CAD build for the part. Positions are in the model's coordinates, mm. A direction names the side the tool comes from. Give positions to 0.01 mm unless a question says otherwise; leave off trailing zeros. Loops run counter-clockwise (first coordinate to the right, second up) from the corner with the lowest first, then second, coordinate; pieces in that order, holes last. Notation, with made-up numbers: M 7.25,28.25 L 51.25,28.25 A27 ccw 51.25,56.25 Z; hole C 18.5,89 d6. An arc over 180 degrees is marked long. One line per question, with ' | ' between items.
Autodesk Inventor part; units mm, degrees
ref_plane "Work Plane2" through (0, 0, 2.5) normal (0, 0, 1) x (1, 0, 0)
ref_plane "Work Plane8" through (0, 0, 0) normal (0.9238795, 0.3826834, 0) x (0, 0, 1)
ref_plane "Work Plane9" through (0, 0, 0) normal (1, 0, 0) x (0, 1, 0)
sketch "Sketch1" plane through (0, 0, 0) normal (0, 0, 1) x (1, 0, 0)
  circle A0 centre (0, 0) radius 10
  dimension "d0" = 20
extrude "Extrusion1" add sketch "Sketch1" along normal blind 5
ref_plane "Work Plane2" through (0, 0, 2.5) normal (0, 0, 1) x (1, 0, 0)
sketch "Sketch2" plane through (0, 0, 0) normal (0, 0, -1) x (-1, 0, 0)
  circle A0 centre (0, 0) radius 10
  circle A1 centre (0, 0) radius 8
  dimension "d3" = 16
surface extrude "Pitch Diameter" sketch "Sketch2" against normal through all shown no curves A1
ref_plane "Work Plane8" through (0, 0, 0) normal (0.9238795, 0.3826834, 0) x (0, 0, 1)
ref_plane "Work Plane9" through (0, 0, 0) normal (1, 0, 0) x (0, 1, 0)
spur gear teeth "Spur Gear" teeth 8 pitch diameter 16 tip diameter 20 root diameter 11 face width 5 start plane through (0, 0, 0) normal (0, 0, -1) x (-1, 0, 0)
sketch "Sketch3" plane through (0, 0, 5) normal (0, 0, 1) x (1, 0, 0)
  line L0 (-1.15, 1.185) -> (-1.15, -1.185)
  arc A0 (-1.15, -1.185) -> (-1.15, 1.185) centre (0, 0) ccw
  point P0 (-1.15, 0)
  dimension "d49" = 2.37
  dimension "d50" = 1.15
extrude "Extrusion2" cut sketch "Sketch3" against normal through all
equation "\"d0\" = da_da"
equation "\"d1\" = da_b"
equation "\"d3\" = da_d"
equation "\"d16\" = da_aw"
equation "\"d43\" = da_aw"
equation "\"d46\" = da_aw"
properties part number "Spur Gear1" material "Steel"
Item 1: Mould opens along X. For faces 1 (the cylindrical face through (-6.55, -4.31, 2.46)), 2 (the cylindrical face through (4.257, 6.511, 2.465)), 3 (the flat face through (0, -2, 5)) say: pulls with the +X half, pulls with the -X half, needs draft (parallel to the pull), parting line crosses it, or undercut.
Conclusion:
face 1: pulls with the -X half | face 2: undercut | face 3: needs draft
Item 2: Drill centre lines: line 1 along X through (y, z) = (0, 3.35); line 2 along Y through (x, z) = (0, 3); line 3 along X through (y, z) = (-6.5, 3.6). Where is each one in solid material? Low to high. Write a range as [from, to].
Conclusion:
line 1: [-10, -1.15], [1.65, 10] | line 2: [-10, -1.65], [1.65, 10] | line 3: [-7.6, -4.24], [-1.67, 1.67], [4.24, 7.6]
Item 3: Saw through at A-A on x = 0. Give the cut face in (y, z), and give its area (3 significant figures).
Conclusion:
outline: M -10,0 L -1.65,0 L -1.65,5 L -10,5 Z; M 1.65,0 L 10,0 L 10,5 L 1.65,5 Z | area: 83.5 mm²
Item 4: Saw through at D-D on x = 5.75. Give the cut face in (y, z), and give its area (3 significant figures).
Conclusion:
outline: M -7.45,0 L -3.39,0 L -3.39,5 L -7.45,5 Z; M -1.64,0 L 1.64,0 L 1.64,5 L -1.64,5 Z; M 3.39,0 L 7.45,0 L 7.45,5 L 3.39,5 Z | area: 57.1 mm²
Item 5: 3-axis set-ups, long thin cutter, end or side, ignore diameter. For faces 4 (the cylindrical face through (6.511, -4.257, 2.465)), 5 (the cylindrical face through (-4.257, -6.511, 2.465)), 6 (the cylindrical face through (7.614, 1.593, 2.465)): which of +Z, -Z, +X, -X, +Y, -Y reach the whole face in a straight line?
Conclusion:
face 4: +Z, -Z, +X | face 5: +Z, -Z, -Y | face 6: +Z, -Z
Item 6: Saw through at B-B on y = 0. Give the cut face in (x, z).
Conclusion:
outline: M -10,0 L -1.15,0 L -1.15,5 L -10,5 Z; M 1.65,0 L 10,0 L 10,5 L 1.65,5 Z
Item 7: Drop a flat-ended pin along its axis: P1, Ø3, axis at x = 7, z = 2.5, coming from the -Y side. Give the stop position or say it passes through.
Conclusion:
P1: y = -7.73
